Input: part model. Units: mm. Frame: model coordinates. A direction names the side the tool comes from. Coordinates: 2 decimals unless noted, no trailing zeros. Loops run counter-clockwise (first coordinate to the right, second up) from the corner with the lowest first, then second, coordinate; pieces in that order, holes last.
Item 1: Section B-B on z = 14.75. Return loops of the section in (x, y).
Item 2: Section D-D on x = 17. Return loops of the section in (y, z), and give its area (3 significant figures).
Item 3: Section C-C on y = 30. Return loops of the section in (x, z), and give its area (3 significant figures).
Item 4: Reachability of faces 4 (the flat face through (39.2, -9, 2.5)), 5 (the flat face through (-21.5, 0, 14)) from +Z, -Z, +X, -X, +Y, -Y: full face, straight path, thin tool, end or side. Return the list, or none.
Item 5: Ray query, line 1 along Y through (x, z) = (0, 1.2); line 2 along Y through (x, z) = (7.5, 20.5); line 3 along Y through (x, z) = (17, 2.2). Return the intervals inside material, ascending.
Item 6: Pull-direction query (X, two-part tool) for faces 1 (the flat face through (9.032, 26, 3)), 2 (the flat face through (-25.5, 0, 14)), 3 (the flat face through (25.5, 0, 14)); classes: released by +X, released by -X, zero draft, split by the parting line, or undercut.
Item 7: Section A-A on x = 0. Give the number of separate pieces and of enclosed holes in the cut face, and give its area (3 significant figures).
Item 8: Contact query for flat-ended pins moving along their axis: P1, Ø2.5, axis at x = -19.5, z = 1.5, coming from the +Y side; P2, Ø2.5, axis at y = 7.5, z = 3.5, coming from the +X side; P3, Ø6, axis at x = 0.5, z = 13, coming from the +Y side; P4, Ø6, axis at x = 35, y = 6.5, coming from the -Z side. Output: stop coordinate, or through.
```python
from build123d import *

# Parameters (mm, degrees)
SKETCH1_R           = 45
SKETCH1_R_2         = 2.5
SKETCH1_R_3         = 1.5
BOSS_EXTRUDE1_DEPTH = 5
BOSS_EXTRUDE2_DEPTH = 18.5
SKETCH4_R           = 2
CUT_EXTRUDE1_DEPTH  = 10
CUT_EXTRUDE2_DEPTH  = 10
FILLET1_R           = 2


with BuildPart() as part:
    # Sketch1 → Boss-Extrude1 (new body)
    with BuildSketch(Plane.XY):
        Circle(SKETCH1_R)
        Circle(SKETCH1_R_2, mode=Mode.SUBTRACT)
        with Locations((0, 17)):
            Circle(SKETCH1_R_3, mode=Mode.SUBTRACT)
        with Locations((17, 0)):
            Circle(SKETCH1_R_3, mode=Mode.SUBTRACT)
        with Locations((0, -17)):
            Circle(SKETCH1_R_3, mode=Mode.SUBTRACT)
        with Locations((-17, 0)):
            Circle(SKETCH1_R_3, mode=Mode.SUBTRACT)
    extrude(amount=BOSS_EXTRUDE1_DEPTH)

    # Sketch2 → Boss-Extrude2 (add)
    with BuildSketch(Plane.XY.offset(5)):
        Polygon((-25.5, 10), (-25.5, -10), (-25.5, -14), (0, -14), (0, -10), (-21.5, -10), (-21.5, 10), (0, 10), (0, 14), (-25.5, 14), align=None)
    boss_extrude2 = extrude(amount=BOSS_EXTRUDE2_DEPTH)

    # Mirror1: Boss-Extrude2 across plane
    add(boss_extrude2.mirror(Plane(origin=(0, 0, 0), x_dir=(0, 0, 1), z_dir=(1, 0, 0))))

    # Sketch4 → Cut-Extrude1 (cut)
    with BuildSketch(Plane.XY.offset(5)):
        with Locations((0, 30)):
            Circle(SKETCH4_R)
        with Locations((0, -30)):
            Circle(SKETCH4_R)
    extrude(amount=-CUT_EXTRUDE1_DEPTH, mode=Mode.SUBTRACT)

    # Sketch5 → Cut-Extrude2 (cut)
    with BuildSketch(Plane.XY.offset(5)):
        Polygon((29.689632614, 17.695025445), (29.689632614, 0), (41.689632614, 0), (36.7907688, 17.695025445), (27.214994246, 26.948021081), (9.031781892, 36.201016717), (9.031781892, 17.695025445), align=None)
        Polygon((29.689632614, 0), (29.689632614, -17.695025445), (9.031781892, -17.695025445), (9.031781892, -36.201016717), (27.214994246, -26.948021081), (36.7907688, -17.695025445), (41.689632614, 0), align=None)
        Polygon((-29.689632614, -17.695025445), (-29.689632614, 0), (-41.689632614, 0), (-36.7907688, -17.695025445), (-27.214994246, -26.948021081), (-9.031781892, -36.201016717), (-9.031781892, -17.695025445), align=None)
        Polygon((-29.689632614, 0), (-29.689632614, 17.695025445), (-9.031781892, 17.695025445), (-9.031781892, 36.201016717), (-27.214994246, 26.948021081), (-36.7907688, 17.695025445), (-41.689632614, 0), align=None)
    extrude(amount=-CUT_EXTRUDE2_DEPTH, mode=Mode.SUBTRACT)

    # Fillet1
    fillet1_edges = [part.edges().sort_by_distance(p)[0] for p in [
        (9.031781892, -36.201016717, 2.5),
        (9.031781892, -17.695025445, 2.5),
        (29.689632614, -17.695025445, 2.5),
        (-29.689632614, -17.695025445, 2.5),
        (-9.031781892, -17.695025445, 2.5),
        (-9.031781892, -36.201016717, 2.5),
        (-27.214994246, -26.948021081, 2.5),
        (-36.7907688, -17.695025445, 2.5),
        (-41.689632614, 0, 2.5),
        (-36.7907688, 17.695025445, 2.5),
        (-27.214994246, 26.948021081, 2.5),
        (-9.031781892, 36.201016717, 2.5),
        (-9.031781892, 17.695025445, 2.5),
        (-29.689632614, 17.695025445, 2.5),
        (29.689632614, 17.695025445, 2.5),
        (9.031781892, 17.695025445, 2.5),
        (9.031781892, 36.201016717, 2.5),
        (27.214994246, 26.948021081, 2.5),
        (36.7907688, 17.695025445, 2.5),
        (41.689632614, 0, 2.5),
        (36.7907688, -17.695025445, 2.5),
        (27.214994246, -26.948021081, 2.5),
    ]]
    fillet(fillet1_edges, radius=FILLET1_R)


solid = part.part
```
Results found:
1. outline: (-25.5, -14) - (25.5, -14) - (25.5, 14) - (-25.5, 14) - close; hole (-21.5, -10) - (21.5, -10) - (21.5, 10) - (-21.5, 10) - close
2. outline: (-41.67, 0) - (-32.15, 0) - (-32.15, 5) - (-41.67, 5) - close; (-17.7, 0) - (-1.5, 0) - (-1.5, 5) - (-10, 5) - (-10, 23.5) - (-14, 23.5) - (-14, 5) - (-17.7, 5) - close; (1.5, 0) - (17.7, 0) - (17.7, 5) - (14, 5) - (14, 23.5) - (10, 23.5) - (10, 5) - (1.5, 5) - close; (32.15, 0) - (41.67, 0) - (41.67, 5) - (32.15, 5) - close
2. area: 405 mm2
3. outline: (-33.54, 0) - (-21.22, 0) - (-21.22, 5) - (-33.54, 5) - close; (-9.03, 0) - (-2, 0) - (-2, 5) - (-9.03, 5) - close; (2, 0) - (9.03, 0) - (9.03, 5) - (2, 5) - close; (21.22, 0) - (33.54, 0) - (33.54, 5) - (21.22, 5) - close
3. area: 194 mm2
4. face 4: +Z, -Z
4. face 5: +Z
5. line 1: y = -45 to -32, -28 to -18.5, -15.5 to -2.5, 2.5 to 15.5, 18.5 to 28, 32 to 45
5. line 2: y = -14 to -10, 10 to 14
5. line 3: y = -41.67 to -32.15, -17.7 to -1.5, 1.5 to 17.7, 32.15 to 41.67
6. face 1: undercut
6. face 2: released by -X
6. face 3: released by +X
7. separate pieces: 6
7. enclosed holes: 0
7. area: 503 mm2
8. P1: stops at y = 41.13
8. P2: stops at x = 44.56
8. P3: stops at y = 14
8. P4: passes through
